Work out the finished part from the listing and answer in its coordinate system (mm). Give positions to 0.01 mm unless a question says otherwise; leave off trailing zeros. Loops run counter-clockwise (first coordinate to the right, second up) from the corner with the lowest first, then second, coordinate; pieces in that order, holes last. Notation, with made-up numbers: M -29,40 L -18,40 A29 cw -18,68 Z; hole C 23.25,68 d6. An arc over 180 degrees is marked long. Use a Markdown table: item, result.
```python
from build123d import *

# Parameters (mm, degrees)
SKETCH1_W          = 76.2
SKETCH1_H          = 220.098493
BASE_FLANGE1_DEPTH = 1.5875
CUT_EXTRUDE1_REACH = 234.921
SKETCH6_R          = 3.3782
SKETCH7_R          = 9.525
CUT_EXTRUDE2_DEPTH = 233.921245869
HEM1_START         = -220.098493
HEM1_DEPTH         = 220.098493
HEM1_2_DEPTH       = 220.098493


# Read off the part's stored shape, not the designer's step: Hem1
# Sheet-metal steps are written as plain solids
with BuildPart() as part:
    # Sketch1 → Base-Flange1 (new body)
    with BuildSketch(Plane(origin=(0, 0, 0), x_dir=(1, 0, 0), z_dir=(0, 1, 0))):
        with Locations((-38.1, 110.0492465)):
            Rectangle(SKETCH1_W, SKETCH1_H)
    extrude(amount=-BASE_FLANGE1_DEPTH)

    # Sketch6 → Cut-Extrude1 (cut, up to next)
    with BuildSketch(Plane(origin=(0, 0, 0), x_dir=(1, 0, 0), z_dir=(0, 1, 0)), mode=Mode.PRIVATE) as cut_extrude1_sk1:
        with Locations(Location((-57.15, 207.398493, 0), (0, 0, 270))):
            Circle(SKETCH6_R)
    cut_extrude1_tool1 = extrude(cut_extrude1_sk1.sketch, amount=-CUT_EXTRUDE1_REACH, mode=Mode.PRIVATE) & part.part
    # Sketch6 → Cut-Extrude1 (cut, up to next)
    with BuildSketch(Plane(origin=(0, 0, 0), x_dir=(1, 0, 0), z_dir=(0, 1, 0)), mode=Mode.PRIVATE) as cut_extrude1_sk2:
        with Locations(Location((-19.05, 207.398493, 0), (0, 0, 270))):
            Circle(SKETCH6_R)
    cut_extrude1_tool2 = extrude(cut_extrude1_sk2.sketch, amount=-CUT_EXTRUDE1_REACH, mode=Mode.PRIVATE) & part.part
    # Sketch6 → Cut-Extrude1 (cut, up to next)
    with BuildSketch(Plane(origin=(0, 0, 0), x_dir=(1, 0, 0), z_dir=(0, 1, 0)), mode=Mode.PRIVATE) as cut_extrude1_sk3:
        with Locations(Location((-19.05, 107.14228, 0), (0, 0, 270))):
            Circle(SKETCH6_R)
    cut_extrude1_tool3 = extrude(cut_extrude1_sk3.sketch, amount=-CUT_EXTRUDE1_REACH, mode=Mode.PRIVATE) & part.part
    # Sketch6 → Cut-Extrude1 (cut, up to next)
    with BuildSketch(Plane(origin=(0, 0, 0), x_dir=(1, 0, 0), z_dir=(0, 1, 0)), mode=Mode.PRIVATE) as cut_extrude1_sk4:
        with Locations(Location((-57.15, 107.14228, 0), (0, 0, 270))):
            Circle(SKETCH6_R)
    cut_extrude1_tool4 = extrude(cut_extrude1_sk4.sketch, amount=-CUT_EXTRUDE1_REACH, mode=Mode.PRIVATE) & part.part
    add(cut_extrude1_tool1.solids().sort_by_distance((-57.15, 0, -207.398493))[0], mode=Mode.SUBTRACT)
    add(cut_extrude1_tool2.solids().sort_by_distance((-19.05, 0, -207.398493))[0], mode=Mode.SUBTRACT)
    add(cut_extrude1_tool3.solids().sort_by_distance((-19.05, 0, -107.14228))[0], mode=Mode.SUBTRACT)
    add(cut_extrude1_tool4.solids().sort_by_distance((-57.15, 0, -107.14228))[0], mode=Mode.SUBTRACT)

    # Sketch7 → Cut-Extrude2 (cut, through all)
    with BuildSketch(Plane(origin=(0, 0, 0), x_dir=(1, 0, 0), z_dir=(0, 1, 0))):
        with Locations(Location((-38.1, 50.680493, 0), (0, 0, 270))):
            Circle(SKETCH7_R)
    extrude(amount=-CUT_EXTRUDE2_DEPTH, mode=Mode.SUBTRACT)

    # Hem1 outline → Hem1 (cut)
    with BuildSketch(Plane.XY.offset(HEM1_START)):
        with BuildLine():
            ThreePointArc((-74.5625, -1.5875), (-75.70257264, -1.125432101), (-76.199236463, 0))
            Line((-76.199236463, 0), (-76.2, 0))
            Line((-76.2, 0), (-76.2, -1.5875))
            Line((-76.2, -1.5875), (-74.5625, -1.5875))
        make_face()
        with BuildLine():
            ThreePointArc((-0.000763537, 0), (-0.49742736, -1.125432101), (-1.6375, -1.5875))
            Line((-1.6375, -1.5875), (0, -1.5875))
            Line((0, -1.5875), (0, 0))
            Line((0, 0), (-0.000763537, 0))
        make_face()
    extrude(amount=HEM1_DEPTH, mode=Mode.SUBTRACT)

    # Hem1 2 outline → Hem1 2 (add)
    with BuildSketch(Plane.XY.offset(HEM1_START)):
        with BuildLine():
            Line((-66.675, 0.1), (-66.675, 1.6875))
            Line((-66.675, 1.6875), (-74.5625, 1.6875))
            ThreePointArc((-74.5625, 1.6875), (-75.737932101, 1.19007264), (-76.199236463, 0))
            Line((-76.199236463, 0), (-74.5625, 0))
            ThreePointArc((-74.5625, 0), (-74.6125, 0.05), (-74.5625, 0.1))
            Line((-74.5625, 0.1), (-66.675, 0.1))
        make_face()
        with BuildLine():
            ThreePointArc((-1.6375, 0.1), (-1.5875, 0.05), (-1.6375, 0))
            Line((-1.6375, 0), (-0.000763537, 0))
            ThreePointArc((-0.000763537, 0), (-0.462067899, 1.19007264), (-1.6375, 1.6875))
            Line((-1.6375, 1.6875), (-9.525, 1.6875))
            Line((-9.525, 1.6875), (-9.525, 0.1))
            Line((-9.525, 0.1), (-1.6375, 0.1))
        make_face()
    extrude(amount=HEM1_2_DEPTH)


solid = part.part
```
(1) Consider probe 1 along X at (y, z) = (0.25, -180) (3 decimals); probe 2 along Y at (x, z) = (-61, -72); probe 3 along X at (y, z) = (1.1, -91) (3 decimals). Determine where each line is inside the solid, lowest interval first. Write a range as [from, to].
Entries:
| item | result |
|---|---|
| probe 1 | x = [-76.188, -66.675], [-9.525, -0.012] |
| probe 2 | y = [-1.59, 0] |
| probe 3 | x = [-75.819, -66.675], [-9.525, -0.381] |
(2) A cutting plane is placed at B-B (x = -57.15). Write down the section's boundary in (y, z), and give its area (3 significant figures).
Entries:
| item | result |
|---|---|
| outline | M -1.59,-220.1 L 0,-220.1 L 0,-210.78 L -1.59,-210.78 Z; M -1.59,-204.02 L 0,-204.02 L 0,-110.52 L -1.59,-110.52 Z; M -1.59,-103.76 L 0,-103.76 L 0,0 L -1.59,0 Z |
| area | 328 mm² |
(3) A cutting plane is placed at A-A (x = -38.1). Write down the section's boundary in (y, z), and give its area (3 significant figures).
Entries:
| item | result |
|---|---|
| outline | M -1.59,-220.1 L 0,-220.1 L 0,-60.21 L -1.59,-60.21 Z; M -1.59,-41.16 L 0,-41.16 L 0,0 L -1.59,0 Z |
| area | 319 mm² |
(4) Given P1, Ø22, axis at x = -23.5, z = -75.5, coming from the +Y side; P2, Ø1.5, axis at y = -0.5, z = -77, coming from the +X side; P3, Ø1.3, axis at y = 1, z = -116.5, coming from the -X side, each flat-ended and moving along its own axis, determine where each tip first touches the part or whether it passes through.
Entries:
| item | result |
|---|---|
| P1 | stops at y = 0 |
| P2 | stops at x = 0 |
| P3 | stops at x = -76.17 |
(5) The mould has two halves that part along Y. Classify faces 1 (the flat face through (-39, 0, -112)), 2 (the flat face through (-6, 1.688, -112)), 3 (the cylindrical face through (-57.001, -0.783, -210.773)): released by +Y, released by -Y, zero draft, split by the parting line, or undercut.
Entries:
| item | result |
|---|---|
| face 1 | undercut |
| face 2 | released by +Y |
| face 3 | zero draft |
(6) A cutting plane is placed at D-D (x = -26). Write down the section's boundary in (y, z), and give its area (3 significant figures).
Entries:
| item | result |
|---|---|
| outline | M -1.59,-220.1 L 0,-220.1 L 0,0 L -1.59,0 Z |
| area | 349 mm² |
